Autodesk Inventor part; units mm, degrees
ref_plane "YZ Plane" through (0, 0, 0) normal (1, 0, 0) x (0, 1, 0)
ref_plane "XZ Plane" through (0, 0, 0) normal (0, 1, 0) x (-1, 0, 0)
ref_plane "XY Plane" through (0, 0, 0) normal (0, 0, 1) x (1, 0, 0)
sketch "Sketch1" plane through (0, 0, 0) normal (0, 1, 0) x (-1, 0, 0)
  line L0 (50.8, -31.75) -> (-50.8, -31.75)
  line L1 (-50.8, -31.75) -> (-50.8, 31.75)
  line L2 (-50.8, 31.75) -> (50.8, 31.75)
  line L3 (50.8, 31.75) -> (50.8, -31.75)
  line L4 (-57.1863, 0) -> (79.611, 0) construction
  point P0 (0, 0)
  dimension "d0" = 63.5
  dimension "d2" = 101.6
  dimension "d25" = 31.75
  dimension "d36" = 50.8
extrude "Extrusion1" add sketch "Sketch1" along normal blind 2.54
sketch "Sketch2" plane through (0, 0, 0) normal (0, -1, 0) x (1, 0, 0)
  line L0 (-50.8, -31.75) -> (50.8, -31.75)
  line L1 (50.8, -31.75) -> (50.8, 31.75)
  line L2 (50.8, 31.75) -> (-50.8, 31.75)
  line L3 (-50.8, 31.75) -> (-50.8, -31.75)
  circle A0 centre (-43.18, 0) radius 3.175
  circle A1 centre (43.18, 24.13) radius 3.175
  circle A2 centre (43.18, -24.13) radius 3.175
  line L4 (43.18, 24.13) -> (43.18, -24.13) construction
  point P0 (0, 0)
  dimension "d5" = 6.35
  dimension "d6" = 7.62
  dimension "d7" = 6.35
  dimension "d8" = 7.62
  dimension "d9" = 7.62
  dimension "d12" = 6.35
  dimension "d13" = 7.62
  dimension "d26" = 31.75
extrude "Extrusion2" add sketch "Sketch2" along normal blind 2.032 contours A0 | A1 | A2
hole "Hole1" at (43.18, -2.032, 24.13) direction (0, 1, 0) diameter 1.27 end through all
mirror "Mirror1" about plane through (0, 0, 0) normal (0, 0, 1) of "Hole1"
sketch "Sketch4" plane through (-43.18, -2.032, 0) normal (0, -1, 0) x (1, 0, 0)
  circle A0 centre (0, 0) radius 3.175
  point P0 (43.18, 0)
hole "Hole2" at (-43.18, -2.032, 0) direction (0, 1, 0) diameter 1.27 end through all
sketch "Sketch5" plane through (0, 2.54, 0) normal (0, 1, 0) x (1, 0, 0)
  line L0 (-33.9981, 21.59) -> (33.797, 21.59)
  line L1 (33.797, 21.59) -> (33.797, -21.59)
  line L2 (33.797, -21.59) -> (-33.9981, -21.59)
  line L3 (-33.9981, -21.59) -> (-33.9981, 21.59)
  point P0 (0, 0)
extrude "Extrusion3" cut sketch "Sketch5" against normal blind 0.762
fillet "Fillet1" radius 12.7 4 edges at (-50.8, 1.27, 31.75) (50.8, 1.27, 31.75) (50.8, 1.27, -31.75) (-50.8, 1.27, -31.75)
chamfer "Chamfer1" distance 2.032 angle 45 3 edges at (40.005, 0, -24.13) (40.005, 0, 24.13) (-46.355, 0, 0)
equation "\"d6\" = d13"
equation "\"d8\" = d13"
properties part number "sensor_board_base"
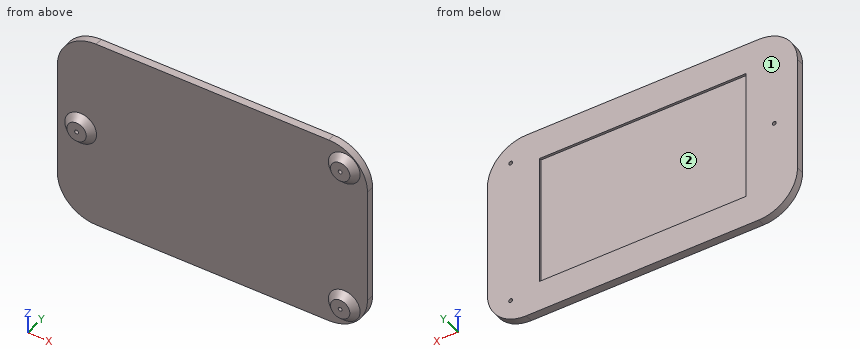
Work out the finished part from the listing and answer in its coordinate system (mm). Face numbers are marked on the shaded views. Round coordinates to 2 decimals unless told otherwise and drop trailing zeros. Write each loop counter-clockwise with the first axis right and the second up, starting at its lowest first coordinate (ties: lowest second). Pieces come first, ordered by that corner, then holes. Notation, with made-up numbers: M 85.5,43.5 L 138.5,43.5 A16 cw 138.5,63.5 Z; hole C 77.25,22.25 d11. An arc over 180 degrees is marked long. Use a Markdown table: item, result.
1) The part is cut by section B-B on z = -11.5. Give the vertices of the cut face in (x, y).
Taken from the geometry:
| item | result |
|---|---|
| outline | M -50.8,0 L 50.8,0 L 50.8,2.54 L 33.8,2.54 L 33.8,1.78 L -34,1.78 L -34,2.54 L -50.8,2.54 Z |
2) Flat-ended cylindrical pins translate along their axes: pin 1 (1.7 mm diameter, centred on x = 43.18, z = 24.13, fed in from +Y); pin 2 (1 mm diameter, centred on x = 43.18, z = -24.13, fed in from +Y); pin 3 (1 mm diameter, centred on x = -26, z = 7, fed in from -Y). Find the tip coordinate at first contact, or state that the pin passes through.
Taken from the geometry:
| item | result |
|---|---|
| pin 1 | stops at y = 2.54 |
| pin 2 | passes through |
| pin 3 | stops at y = 0 |
3) Determine the mould class of the marked faces 1 and 2 for opening direction Z: pulls with the +Z half, pulls with the -Z half, needs draft (parallel to the pull), parting line crosses it, or undercut.
Taken from the geometry:
| item | result |
|---|---|
| face 1 | needs draft |
| face 2 | undercut |
4) The part is cut by section C-C on x = 16. Give the vertices of the cut face in (y, z).
Taken from the geometry:
| item | result |
|---|---|
| outline | M 0,-31.75 L 2.54,-31.75 L 2.54,-21.59 L 1.78,-21.59 L 1.78,21.59 L 2.54,21.59 L 2.54,31.75 L 0,31.75 Z |
5) The part is cut by section A-A on y = -0.85. Give the vertices of the cut face in (x, z) (1 decimal).
Taken from the geometry:
| item | result |
|---|---|
| outline | C -43.2,0 d8.7; C 43.2,-24.1 d8.7; C 43.2,24.1 d8.7; hole C -43.2,0 d1.3; hole C 43.2,-24.1 d1.3; hole C 43.2,24.1 d1.3 |
6) Consider line 1 (Z direction, x = 2.5, y = 2); line 2 (Y direction, x = 10.5, z = 8.5); line 3 (Z direction, x = 43.18, y = 0.8) (3 decimals). Determine where each line is inside the solid, lowest interval first. Write a range as [from, to].
Taken from the geometry:
| item | result |
|---|---|
| line 1 | z = [-31.75, -21.59], [21.59, 31.75] |
| line 2 | y = [0, 1.78] |
| line 3 | z = [-30.69, -24.765], [-23.495, 23.495], [24.765, 30.69] |
